Source: CAD feature listing. Evaluate the final solid. Frame: model axes, mm. A direction names the side the tool comes from. Give positions to 0.01 mm unless a question says otherwise; leave off trailing zeros. Write each loop counter-clockwise with the first axis right and the second up, starting at its lowest first coordinate (ties: lowest second). Pieces come first, ordered by that corner, then holes. Notation, with made-up numbers: (24.5, 14) -> (47.5, 14) arc R21 cw to (47.5, 43) -> close; hole circle Ø3 at (57, 24). An arc over 180 degrees is marked (long way). Answer as a JSON object with one key per item and string values. Group by question number.
Item 1: Ray query, probe 1 along X at (y, z) = (7, 5); probe 2 along Y at (x, z) = (11.75, 22); probe 3 along Y at (x, z) = (14.5, 17.5). Return the intervals inside material, ascending. Write a range as from..to.
Item 2: Pull-direction query (X, two-part tool) for faces 3 (the face through (21.499, 9, 37)), 4 (the face through (6.549, 11, 37)), 5 (the face through (8, 8, 75)); classes: pulls with the +X half, pulls with the -X half, needs draft (parallel to the pull), parting line crosses it, or undercut.
Item 3: First-contact query: pin 1 Ø3 at (x, z) = (4, 33.5) entering from +Y; pin 2 Ø1.3 at (x, z) = (17.5, 29) entering from +Y. Flat tips, straight axial feed; report the tip coordinate or a pass-through.
Item 4: Access query for faces 1 (the face through (0.049, 9, 37)), 2 (the face through (19.549, 11, 37)). Directions: +Z, -Z, +X, -X, +Y, -Y. A direction counts if a zero-diameter tool reaches every point of the face in a straight line with its end or side. Return the directions, or none.
Item 5: Section query A-A on y = 6. Return the cut outline in (x, z), plus the area to 3 significant figures.
from build123d import *

# Parameters (mm, degrees)
BOSS_EXTRUDE1_DEPTH = 75


with BuildPart() as part:
    # Model → Boss-Extrude1 (new body)
    with BuildSketch(Plane.XY):
        with BuildLine():
            Line((12.048720141, 3), (10.773720141, 3))
            Line((10.773720141, 3), (9.498720141, 3))
            ThreePointArc((9.498720141, 3), (8.79161336, 3.292893219), (8.498720141, 4))
            Line((8.498720141, 4), (8.498720141, 18.3))
            ThreePointArc((8.498720141, 18.3), (8.293694888, 18.794974747), (7.798720141, 19))
            Line((7.798720141, 19), (7.248720141, 19))
            ThreePointArc((7.248720141, 19), (6.753745394, 18.794974747), (6.548720141, 18.3))
            Line((6.548720141, 18.3), (6.548720141, 4))
            ThreePointArc((6.548720141, 4), (6.255826922, 3.292893219), (5.548720141, 3))
            Line((5.548720141, 3), (2.998720141, 3))
            ThreePointArc((2.998720141, 3), (2.29161336, 3.292893219), (1.998720141, 4))
            Line((1.998720141, 4), (1.998720141, 18.3))
            ThreePointArc((1.998720141, 18.3), (1.793694888, 18.794974747), (1.298720141, 19))
            Line((1.298720141, 19), (0.748720141, 19))
            ThreePointArc((0.748720141, 19), (0.253745394, 18.794974747), (0.048720141, 18.3))
            Line((0.048720141, 18.3), (0.048720141, 0))
            Line((0.048720141, 0), (10.773720141, 0))
            Line((10.773720141, 0), (21.498720141, 0))
            Line((21.498720141, 0), (21.498720141, 18.3))
            ThreePointArc((21.498720141, 18.3), (21.293694888, 18.794974747), (20.798720141, 19))
            Line((20.798720141, 19), (20.248720141, 19))
            ThreePointArc((20.248720141, 19), (19.753745394, 18.794974747), (19.548720141, 18.3))
            Line((19.548720141, 18.3), (19.548720141, 4))
            ThreePointArc((19.548720141, 4), (19.255826922, 3.292893219), (18.548720141, 3))
            Line((18.548720141, 3), (15.998720141, 3))
            ThreePointArc((15.998720141, 3), (15.29161336, 3.292893219), (14.998720141, 4))
            Line((14.998720141, 4), (14.998720141, 18.3))
            ThreePointArc((14.998720141, 18.3), (14.793694888, 18.794974747), (14.298720141, 19))
            Line((14.298720141, 19), (13.748720141, 19))
            ThreePointArc((13.748720141, 19), (13.253745394, 18.794974747), (13.048720141, 18.3))
            Line((13.048720141, 18.3), (13.048720141, 4))
            ThreePointArc((13.048720141, 4), (12.755826922, 3.292893219), (12.048720141, 3))
        make_face()
    extrude(amount=BOSS_EXTRUDE1_DEPTH)


solid = part.part
Worked answers:
{
 "1": {"probe 1": "0.05..2, 6.55..8.5, 13.05..15, 19.55..21.5", "probe 2": "0..3", "probe 3": "0..18.97"},
 "2": {"face 3": "pulls with the +X half", "face 4": "undercut", "face 5": "needs draft"},
 "3": {"pin 1": "y = 3.13", "pin 2": "y = 3"},
 "4": {"face 1": "+Z, -Z, -X, +Y, -Y", "face 2": "+Z, -Z, +Y"},
 "5": {"outline": "(0.05, 0) -> (2, 0) -> (2, 75) -> (0.05, 75) -> close; (6.55, 0) -> (8.5, 0) -> (8.5, 75) -> (6.55, 75) -> close; (13.05, 0) -> (15, 0) -> (15, 75) -> (13.05, 75) -> close; (19.55, 0) -> (21.5, 0) -> (21.5, 75) -> (19.55, 75) -> close", "area": "585 mm^2"}
}
